Can you work these out from the model? Positions are in its coordinate system, mm. Face numbers are marked on the shaded views. Round coordinates to 2 decimals unless told otherwise and drop trailing zeros. Write each loop counter-clockwise with the first axis right and the second up, starting at its lowest first coordinate (ties: lowest second). Pieces come first, ordered by that corner, then holes. Notation, with made-up numbers: (-8, -0.75) -> (46, -0.75) arc R11 ccw to (46, 4.25) -> close; hole circle Ø11 at (76.5, -0.75). An arc over 180 degrees is marked (long way). Write item = value, one per line. Start each with the question number.
1) Imagine slicing it at A-A, the plane y = 7. Please give me the cut outline in (x, z), then the cut area to 3 significant figures.
2) Imagine slicing it at D-D, the plane y = 26.5. Please give me the cut outline in (x, z), then the cut area to 3 significant figures.
3) Thinking about a two-plate mould opening in X: for the marked faces 1, 2 and 3, which applies, +X half, -X half, draft (parallel to the pull), parting line (faces both ways), or undercut?
4) I'm going to push flat-ended pins straight in: pin 1 (8 mm diameter, centred on x = 28.5, z = 3.5, fed in from +Y); pin 2 (1.5 mm diameter, centred on x = -18, z = 6.5, fed in from +Y); pin 3 (1.6 mm diameter, centred on x = -17, y = -5.5, fed in from +Z). Where does each tip first touch, or does it pass through?
5) Imagine slicing it at B-B, the plane x = -17.5. Please give me the cut outline in (y, z) (3 decimals).
6) Imagine slicing it at C-C, the plane z = -7.75. Please give me the cut outline in (x, y) (3 decimals).
7) If I drill on line 1 (Y direction, x = -50, z = 4.75) (3 decimals); line 2 (X direction, y = 19.5, z = -8); line 3 (Y direction, x = 49, z = -0.25) (3 decimals), over which ranges is the centre line in solid material (lowest first)?
from build123d import *

# Parameters (mm, degrees)
BOSS_EXTRUDE1_DEPTH      = 10
BOSS_EXTRUDE1_DEPTH_BACK = 10
SKETCH2_W                = 4.8
SKETCH2_H                = 4.8
SKETCH2_W_2              = 3.2
BOSS_EXTRUDE2_DEPTH      = 10
CUT_EXTRUDE1_DEPTH       = 5.2


with BuildPart() as part:
    # Sketch1 → Boss-Extrude1 (new, two sides: drawn at the far end of the back side and taken through both)
    with BuildSketch(Plane.XY.offset(-BOSS_EXTRUDE1_DEPTH_BACK)):
        Polygon((-55, 21.875), (55, -5.625), (55, -8.125), (-55, -8.125), align=None)
    extrude(amount=BOSS_EXTRUDE1_DEPTH + BOSS_EXTRUDE1_DEPTH_BACK)

    # Sketch2 → Boss-Extrude2 (add)
    with BuildSketch(Plane(origin=(1.911764706, 7.647058824, 0), x_dir=(0.970142500145332, -0.24253562503633289, 0), z_dir=(0.24253562503633289, 0.970142500145332, 0))):
        with Locations((-51.063304306, 7.6)):
            Rectangle(SKETCH2_W, SKETCH2_H)
        with Locations((-51.863304306, -7.6)):
            Rectangle(SKETCH2_W_2, SKETCH2_H)
        with Locations((18.686695694, -7.6)):
            Rectangle(SKETCH2_W_2, SKETCH2_H)
        with Locations((17.886695694, 7.6)):
            Rectangle(SKETCH2_W, SKETCH2_H)
    extrude(amount=BOSS_EXTRUDE2_DEPTH)

    # Sketch3 → Cut-Extrude1 (cut)
    with BuildSketch(Plane.XZ.offset(8.125)):
        Polygon((15.692093342, -10.058542854), (14.11294757, -4.9), (22.553719096, -4.9), (20.974573324, -10.058542854), align=None)
        Polygon((-20.974573324, -10.058542854), (-22.553719096, -4.9), (-14.11294757, -4.9), (-15.692093342, -10.058542854), align=None)
        Polygon((-20.974573324, 10.058542854), (-22.553719096, 4.9), (-14.11294757, 4.9), (-15.692093342, 10.058542854), align=None)
        Polygon((15.692093342, 10.058542854), (14.11294757, 4.9), (22.553719096, 4.9), (20.974573324, 10.058542854), align=None)
    extrude(amount=-CUT_EXTRUDE1_DEPTH, mode=Mode.SUBTRACT)


solid = part.part
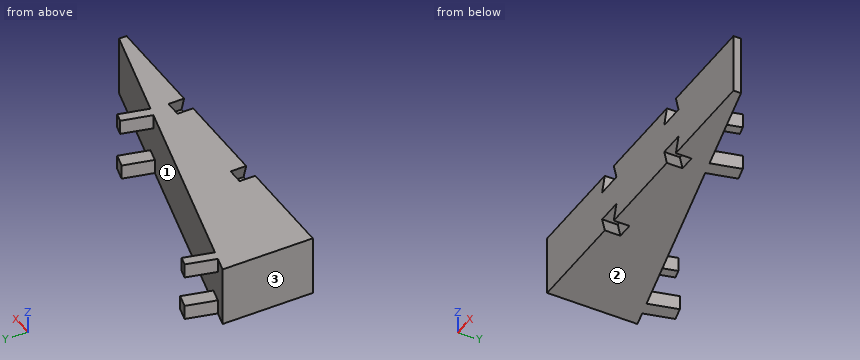
Reported:
q1.outline = (-55, -10) -> (4.5, -10) -> (4.5, 10) -> (-55, 10) -> close; (17.71, -10) -> (22.66, -10) -> (22.66, -5.2) -> (17.71, -5.2) -> close; (19.36, 5.2) -> (22.66, 5.2) -> (22.66, 10) -> (19.36, 10) -> close
q1.area = 1,230 mm²
q2.outline = (-48.48, -10) -> (-43.54, -10) -> (-43.54, -5.2) -> (-48.48, -5.2) -> close; (-48.48, 5.2) -> (-45.19, 5.2) -> (-45.19, 10) -> (-48.48, 10) -> close
q2.area = 39.6 mm²
q3.face_1 = undercut
q3.face_2 = draft
q3.face_3 = -X half
q4.pin_1 = 2
q4.pin_2 = 12.81
q4.pin_3 = 4.9
q5.outline = (-8.125, -4.9) -> (-2.925, -4.9) -> (-2.925, -10) -> (12.5, -10) -> (12.5, 10) -> (-2.925, 10) -> (-2.925, 4.9) -> (-8.125, 4.9) -> close
q6.outline = (-55, -8.125) -> (-21.681, -8.125) -> (-21.681, -2.925) -> (-14.985, -2.925) -> (-14.985, -8.125) -> (14.985, -8.125) -> (14.985, -2.925) -> (21.681, -2.925) -> (21.681, -8.125) -> (55, -8.125) -> (55, -5.625) -> (21.593, 2.727) -> (24.018, 12.428) -> (19.361, 13.592) -> (16.936, 3.891) -> (-45.299, 19.45) -> (-42.873, 29.151) -> (-47.53, 30.315) -> (-49.955, 20.614) -> (-55, 21.875) -> close
q7.line_1 = -8.125 to 20.625
q7.line_2 = -55 to -45.29
q7.line_3 = -8.125 to -4.125
